Geometry check sheet. Reference: the model listing, model coordinates, mm. Face numbers are marked on the shaded views. A direction names the side the tool comes from. Round coordinates to 2 decimals unless told otherwise and drop trailing zeros. Loops run counter-clockwise (first coordinate to the right, second up) from the corner with the lowest first, then second, coordinate; pieces in that order, holes last. Notation, with made-up numbers: (-6.75, 61) -> (9.25, 61) arc R21 ccw to (9.25, 93) -> close; hole circle Ø5 at (63, 17). An arc over 180 degrees is marked (long way). Use one line per item in the form item = value.
from build123d import *

# Parameters (mm, degrees)
SKETCH2_R           = 18.9
BOSS_EXTRUDE1_DEPTH = 5
SKETCH2_4_R         = 17.9
CUT_EXTRUDE1_DEPTH  = 3.95
SKETCH7_R           = 12.8
BOSS_EXTRUDE2_DEPTH = 2.5
SKETCH8_R           = 13.95
BOSS_EXTRUDE3_DEPTH = 2.5


with BuildPart() as part:
    # Sketch2 → Boss-Extrude1 (new body)
    with BuildSketch(Plane(origin=(0, 0, 0), x_dir=(0, 0, -1), z_dir=(1, 0, 0))):
        Circle(SKETCH2_R)
    extrude(amount=BOSS_EXTRUDE1_DEPTH)

    # Sketch2<4> → Cut-Extrude1 (cut)
    with BuildSketch(Plane(origin=(0, 0, 0), x_dir=(0, 0, -1), z_dir=(1, 0, 0))):
        Circle(SKETCH2_4_R)
    extrude(amount=CUT_EXTRUDE1_DEPTH, mode=Mode.SUBTRACT)

    # Sketch7 → Boss-Extrude2 (add)
    with BuildSketch(Plane(origin=(5, 0, 0), x_dir=(0, 0, -1), z_dir=(1, 0, 0))):
        Circle(SKETCH7_R)
    extrude(amount=BOSS_EXTRUDE2_DEPTH)

    # Sketch8 → Boss-Extrude3 (add)
    with BuildSketch(Plane(origin=(7.5, 0, 0), x_dir=(0, 0, -1), z_dir=(1, 0, 0))):
        Circle(SKETCH8_R)
    extrude(amount=BOSS_EXTRUDE3_DEPTH)


solid = part.part
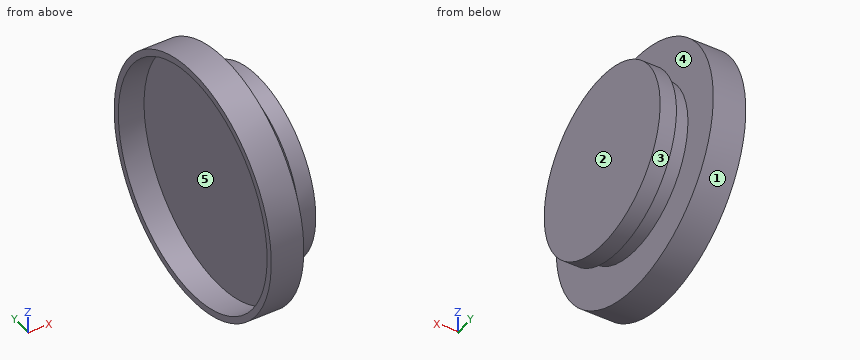
1. Gauge pin test, flat ends, axial feed: pin 1 (2 mm diameter, centred on x = 1.5, y = 15, fed in from -Z); pin 2 (14 mm diameter, centred on y = 4, z = -3, fed in from -X); pin 3 (4 mm diameter, centred on x = 3.5, y = 9, fed in from -Z). Record the tip position at first contact, or that the pin passes through.
Return value:
pin_1 = -12.7
pin_2 = 3.95
pin_3 = -17.56
2. Material ranges on line 1 along Y through (x, z) = (2.35, 0); line 2 along Y through (x, z) = (4.75, 0); line 3 along X through (y, z) = (-10.5, 11), recorded low to high.
Return value:
line_1 = -18.9 to -17.9, 17.9 to 18.9
line_2 = -18.9 to 18.9
line_3 = 3.95 to 5
3. Section check D-D (x = 6.75). Record the boundary of the cut face in (y, z).
Return value:
outline = circle Ø25.6 at (0, 0)
4. Section check B-B (x = 1.25). Record the boundary of the cut face in (y, z), then the cut area to 3 significant figures.
Return value:
outline = circle Ø37.8 at (0, 0); hole circle Ø35.8 at (0, 0)
area = 116 mm2
5. Section check A-A (z = 0). Record the boundary of the cut face in (x, y), then the cut area to 3 significant figures.
Return value:
outline = (0, -18.9) -> (5, -18.9) -> (5, -12.8) -> (7.5, -12.8) -> (7.5, -13.95) -> (10, -13.95) -> (10, 13.95) -> (7.5, 13.95) -> (7.5, 12.8) -> (5, 12.8) -> (5, 18.9) -> (0, 18.9) -> (0, 17.9) -> (3.95, 17.9) -> (3.95, -17.9) -> (0, -17.9) -> close
area = 181 mm2
6. Tool access check on the marked faces 1, 2, 3, 4 and 5. Record the directions out of +Z, -Z, +X, -X, +Y, -Y that give a thin tool (end or side, any length) a straight path to the whole face; none if there is none.
Return value:
face_1 = +X, -X
face_2 = +Z, -Z, +X, +Y, -Y
face_3 = +X
face_4 = none
face_5 = -X
